Design review of the part built by this model. Coordinates are the model's own, in mm. Coordinates: 2 decimals unless noted, no trailing zeros. Write each loop counter-clockwise with the first axis right and the second up, starting at its lowest first coordinate (ties: lowest second). Pieces come first, ordered by that corner, then holes.
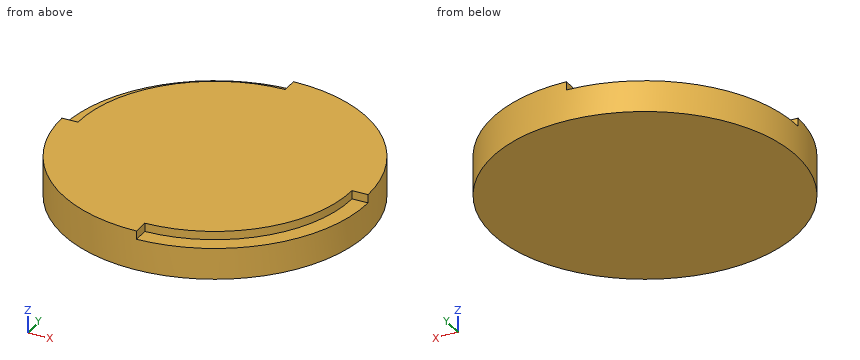
```python
from build123d import *

# Parameters (mm, degrees)
F0_R     = 20
F0_R_2   = 10.1
F1_DEPTH = 2
F2_DEPTH = 4.2
F3_R     = 20
F3_R_2   = 10.1
F4_DEPTH = 1
F6_DEPTH = 1.1


with BuildPart() as f1:
    # F0 (on Top) → F1 (new body)
    with BuildSketch(Plane.XY):
        Circle(F0_R)
        Circle(F0_R_2, mode=Mode.SUBTRACT)
        Circle(F0_R_2)
    extrude(amount=F1_DEPTH)

    # F0 (on Top) → F2 (join)
    with BuildSketch(Plane.XY):
        Circle(F0_R)
        Circle(F0_R_2, mode=Mode.SUBTRACT)
    extrude(amount=F2_DEPTH)

    # F3 (on face) → F4 (join)
    with BuildSketch(Plane.XY.offset(4.2)):
        Circle(F3_R)
        Circle(F3_R_2, mode=Mode.SUBTRACT)
        Circle(F3_R_2)
    extrude(amount=F4_DEPTH)

    # F5 (on face) → F6 (cut)
    with BuildSketch(Plane.XY.offset(5.2)):
        with BuildLine():
            ThreePointArc((0, 20), (-14.1421356237, 14.1421356237), (-20, 0))
            Line((-20, 0), (-17.9, 0))
            ThreePointArc((-17.9, 0), (-12.6572113832, 12.6572113832), (0, 17.9))
            Line((0, 17.9), (0, 20))
        make_face()
        with BuildLine():
            Line((0, -17.9), (0, -20))
            ThreePointArc((0, -20), (14.1421356237, -14.1421356237), (20, 0))
            Line((20, 0), (17.9, 0))
            ThreePointArc((17.9, 0), (12.6572113832, -12.6572113832), (0, -17.9))
        make_face()
    extrude(amount=-F6_DEPTH, mode=Mode.SUBTRACT)


solid = f1.part
```
(1) Wall thickness on line 1 (Z direction, x = 1, y = 8.5); line 2 (Y direction, x = 0, z = 3); line 3 (Z direction, x = 18.5, y = -1): over which ranges is each line inside the solid? List them lowest first.
(2) Insertion check: pin 1 Ø3 at (y, z) = (4, 1) entering from -X; pin 2 Ø3 at (y, z) = (15, 4) entering from +X; pin 3 Ø3 at (y, z) = (-7, 3.5) entering from -X. Each pin has a flat end and moves straight along its axis. Give the tip position at first contact, or say it passes through.
(3) Consider section C-C (x = -5). Give the boundary of the cut face in (y, z), plus the area to 3 significant figures.
(4) Consider section B-B (y = 2). Give the boundary of the cut face in (x, z), plus the area to 3 significant figures.
(5) Consider section D-D (x = 16). Give the boundary of the cut face in (y, z), plus the area to 3 significant figures.
(6) Consider section A-A (z = 4.7). Give the boundary of the cut face in (x, y), plus the area to 3 significant figures.
Results:
1. line 1: z = 0 to 2, 4.2 to 5.2
1. line 2: y = -20 to -10.1, 10.1 to 20
1. line 3: z = 0 to 4.1
2. pin 1: stops at x = -19.84
2. pin 2: stops at x = 14.76
2. pin 3: stops at x = -19.23
3. outline: (-19.36, 0) - (19.36, 0) - (19.36, 4.1) - (17.19, 4.1) - (17.19, 5.2) - (-19.36, 5.2) - close; hole (-8.78, 2) - (8.78, 2) - (8.78, 4.2) - (-8.78, 4.2) - close
3. area: 160 mm2
4. outline: (-19.9, 0) - (19.9, 0) - (19.9, 5.2) - (-17.79, 5.2) - (-17.79, 4.1) - (-19.9, 4.1) - close; hole (-9.9, 2) - (9.9, 2) - (9.9, 4.2) - (-9.9, 4.2) - close
4. area: 161 mm2
5. outline: (-12, 0) - (12, 0) - (12, 5.2) - (-8.03, 5.2) - (-8.03, 4.1) - (-12, 4.1) - close
5. area: 120 mm2
6. outline: (-20, 0) arc R20 ccw to (0, -20) - (0, -17.9) arc R17.9 ccw to (17.9, 0) - (20, 0) arc R20 ccw to (0, 20) - (0, 17.9) arc R17.9 ccw to (-17.9, 0) - close
6. area: 1,130 mm2
